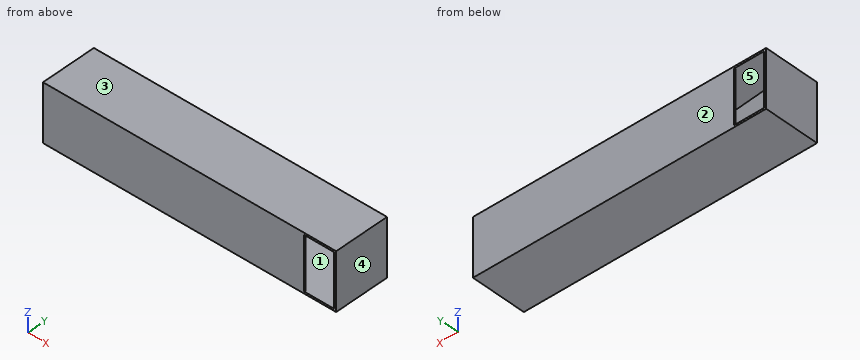
from build123d import *

# Parameters (mm, degrees)
ESQUISSE1_W             = 743.48850074
ESQUISSE1_H             = 139.522790213
ESQUISSE1_W_2           = 733.48850074
ESQUISSE1_H_2           = 133.522790213
BOSS_EXTRU_1_DEPTH      = 135
ESQUISSE1_4_W           = 743.48850074
ESQUISSE1_4_H           = 139.522790213
ESQUISSE1_4_W_2         = 733.48850074
ESQUISSE1_4_H_2         = 133.522790213
BOSS_EXTRU_3_DEPTH      = 5
ESQUISSE2_W             = 743.48850074
ESQUISSE2_H             = 139.522790213
BOSS_EXTRU_4_DEPTH      = 5
ESQUISSE3_W             = 76
ESQUISSE3_H             = 135
ENL_V_MAT_EXTRU_1_DEPTH = 10
ESQUISSE4_W             = 76
ESQUISSE4_H             = 135
ENL_V_MAT_EXTRU_2_DEPTH = 10


with BuildPart() as part:
    # Esquisse1 → Boss.-Extru.1 (new body)
    # profile 1 of 2: a face of its own
    with BuildSketch(Plane.XY):
        with Locations((335.166692979, 135.809178026)):
            Rectangle(ESQUISSE1_W, ESQUISSE1_H)
        with Locations((335.166692979, 135.809178026)):
            Rectangle(ESQUISSE1_W_2, ESQUISSE1_H_2, mode=Mode.SUBTRACT)
    # profile 2 of 2: a face of its own
    with BuildSketch(Plane.XY):
        Polygon((625.910943349, 69.047782919), (-31.577557391, 126.570573132), (-31.577557391, 121.551473945), (568.542377121, 69.047782919), align=None)
    extrude(amount=BOSS_EXTRU_1_DEPTH)

    # Esquisse1_4 → Boss.-Extru.3 (add)
    # profile 1 of 4: a face of its own
    with BuildSketch(Plane.XY):
        with Locations((335.166692979, 135.809178026)):
            Rectangle(ESQUISSE1_4_W, ESQUISSE1_4_H)
        with Locations((335.166692979, 135.809178026)):
            Rectangle(ESQUISSE1_4_W_2, ESQUISSE1_4_H_2, mode=Mode.SUBTRACT)
    # profile 2 of 4: a face of its own
    with BuildSketch(Plane.XY):
        Polygon((625.910943349, 69.047782919), (-31.577557391, 126.570573132), (-31.577557391, 121.551473945), (568.542377121, 69.047782919), align=None)
    # profile 3 of 4: a face of its own
    with BuildSketch(Plane.XY):
        Polygon((568.542377121, 69.047782919), (-31.577557391, 121.551473945), (-31.577557391, 69.047782919), align=None)
    # profile 4 of 4: a face of its own
    with BuildSketch(Plane.XY):
        Polygon((-31.577557391, 202.570573132), (-31.577557391, 126.570573132), (625.910943349, 69.047782919), (701.910943349, 69.047782919), (701.910943349, 202.570573132), align=None)
    extrude(amount=-BOSS_EXTRU_3_DEPTH)

    # Esquisse2 → Boss.-Extru.4 (add)
    with BuildSketch(Plane.XY.offset(135)):
        with Locations((335.166692979, 135.809178026)):
            Rectangle(ESQUISSE2_W, ESQUISSE2_H)
    extrude(amount=BOSS_EXTRU_4_DEPTH)

    # Esquisse3 → Enl_v. mat.-Extru.1 (cut)
    with BuildSketch(Plane(origin=(0, 205.570573132, 0), x_dir=(1, 0, 0), z_dir=(0, 1, 0))):
        with Locations((6.422442609, -67.5)):
            Rectangle(ESQUISSE3_W, ESQUISSE3_H)
    extrude(amount=-ENL_V_MAT_EXTRU_1_DEPTH, mode=Mode.SUBTRACT)

    # Esquisse4 → Enl_v. mat.-Extru.2 (cut)
    with BuildSketch(Plane.XZ.offset(-66.047782919)):
        with Locations((663.910943349, 67.5)):
            Rectangle(ESQUISSE4_W, ESQUISSE4_H)
    extrude(amount=-ENL_V_MAT_EXTRU_2_DEPTH, mode=Mode.SUBTRACT)


solid = part.part
Read the model definition and answer for the solid it produces. Units are mm, in the model's axes. Face numbers are marked on the shaded views. A direction names the side the tool comes from. Coordinates: 2 decimals unless noted, no trailing zeros. Loops run counter-clockwise (first coordinate to the right, second up) from the corner with the lowest first, then second, coordinate; pieces in that order, holes last. Notation, with made-up numbers: (57, 75.5) -> (69, 75.5) arc R29 ccw to (69, 113.5) -> close; hole circle Ø7 at (-29, -31.75). An arc over 180 degrees is marked (long way). Answer in a Markdown table with one row per item.
Item 1: For a pull along Y with two mould halves and no side action, classify the marked faces 1, 2 and 3 as released by +Y, released by -Y, zero draft, split by the parting line, or undercut.
Returned:
| item | result |
|---|---|
| face 1 | undercut |
| face 2 | released by +Y |
| face 3 | zero draft |
Item 2: A cutting plane is placed at D-D on y = 75.5. Determine the outline of the cut face in (x, z).
Returned:
| item | result |
|---|---|
| outline | (-36.58, -5) -> (706.91, -5) -> (706.91, 140) -> (-36.58, 140) -> close; hole (-31.58, 0) -> (494.79, 0) -> (494.79, 135) -> (-31.58, 135) -> close; hole (552.16, 0) -> (701.91, 0) -> (701.91, 135) -> (552.16, 135) -> close |
Item 3: Straight lines are drawn through the part: line 1 along Z through (x, y) = (350.5, 79); line 2 along X through (y, z) = (129, 10); line 3 along Y through (x, z) = (73.5, 106). For each, find the intervals that lie inside material, in ascending order. Write a range as [from, to].
Returned:
| item | result |
|---|---|
| line 1 | z = [-5, 0], [135, 140] |
| line 2 | x = [-36.58, -31.58], [701.91, 706.91] |
| line 3 | y = [66.05, 69.05], [112.36, 117.38], [202.57, 205.57] |
Item 4: For the marked faces 4 and 5, determine the directions among +Z, -Z, +X, -X, +Y, -Y from which every point of the face is accessible in a straight line to the end or side of a thin tool.
Returned:
| item | result |
|---|---|
| face 4 | +Z, -Z, +X, +Y, -Y |
| face 5 | none |
Item 5: A cutting plane is placed at A-A on z = 90. Determine the outline of the cut face in (x, y).
Returned:
| item | result |
|---|---|
| outline | (-36.58, 66.05) -> (625.91, 66.05) -> (625.91, 69.05) -> (-31.58, 126.57) -> (-31.58, 205.57) -> (-36.58, 205.57) -> close; (44.42, 202.57) -> (701.91, 202.57) -> (701.91, 66.05) -> (706.91, 66.05) -> (706.91, 205.57) -> (44.42, 205.57) -> close; hole (-31.58, 69.05) -> (568.54, 69.05) -> (-31.58, 121.55) -> close |
Item 6: A cutting plane is placed at C-C on x = 495. Determine the outline of the cut face in (y, z).
Returned:
| item | result |
|---|---|
| outline | (66.05, -5) -> (205.57, -5) -> (205.57, 140) -> (66.05, 140) -> close; hole (69.05, 0) -> (75.48, 0) -> (75.48, 135) -> (69.05, 135) -> close; hole (80.5, 0) -> (202.57, 0) -> (202.57, 135) -> (80.5, 135) -> close |
Item 7: A cutting plane is placed at B-B on y = 193. Determine the outline of the cut face in (x, z).
Returned:
| item | result |
|---|---|
| outline | (-36.58, -5) -> (706.91, -5) -> (706.91, 140) -> (-36.58, 140) -> close; hole (-31.58, 0) -> (701.91, 0) -> (701.91, 135) -> (-31.58, 135) -> close |
